Check sheet for the modelled part. Datum: model origin and axes. Units: mm. Face numbers are marked on the shaded views. A direction names the side the tool comes from. Coordinates: 2 decimals unless noted, no trailing zeros. Loops run counter-clockwise (first coordinate to the right, second up) from the corner with the lowest first, then second, coordinate; pieces in that order, holes last. Notation, with made-up numbers: (46.5, 41) - (91.5, 41) arc R9 ccw to (91.5, 46) - close; hole circle Ø11 at (78, -34). An arc over 180 degrees is marked (long way). Use a Markdown table: item, result. Add a question column.
1) Sectioned sample at B-B, the plane y = 7.5. Enter the section's corners in (x, z).
2) Thickness scan on line 1 (Z direction, x = 3.5, y = -6.25); line 2 (Y direction, x = -0.25, z = 61); line 3 (Z direction, x = 1.5, y = 1.75). Record the ranges inside material, lowest first.
3) Tool access check on the marked faces 1 and 2. Record the directions out of +Z, -Z, +X, -X, +Y, -Y that give a thin tool (end or side, any length) a straight path to the whole face; none if there is none.
4) Go/stop test with flat-tipped pins: P1, Ø1.5, axis at x = 2, y = 4, coming from the -Z side; P2, Ø6, axis at y = -1.5, z = 55, coming from the -X side. Record where each tip stops, or that it passes through.
5) Sectioned sample at A-A, the plane z = 31. Enter the section's corners in (x, y).
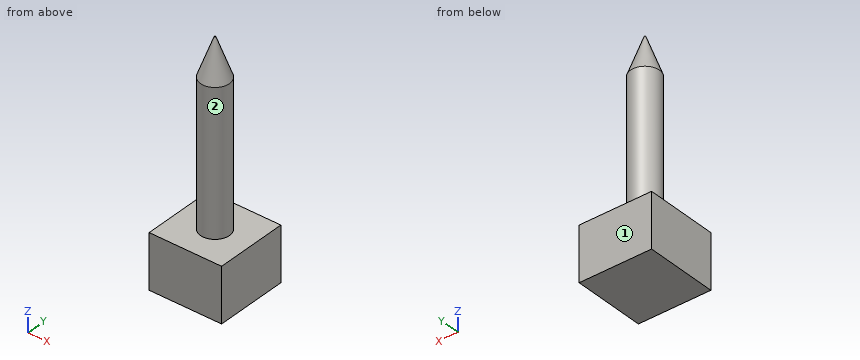
from build123d import *

# Parameters (mm, degrees)
SKETCH1_W           = 20
SKETCH1_H           = 20
BOSS_EXTRUDE1_DEPTH = 15
SKETCH2_R           = 4
BOSS_EXTRUDE2_DEPTH = 50
CHAMFER1_SIZE       = 10.5
CHAMFER1_SIZE2      = 3.82168746


with BuildPart() as part:
    # Sketch1 → Boss-Extrude1 (new body)
    with BuildSketch(Plane.XY):
        Rectangle(SKETCH1_W, SKETCH1_H)
    extrude(amount=BOSS_EXTRUDE1_DEPTH)

    # Sketch2 → Boss-Extrude2 (add)
    with BuildSketch(Plane.XY.offset(15)):
        Circle(SKETCH2_R)
    extrude(amount=BOSS_EXTRUDE2_DEPTH)

    # Chamfer1
    chamfer1_edges = [part.edges().sort_by_distance(p)[0] for p in [
        (-4, 0, 65),
    ]]
    chamfer1_side = [part.faces().sort_by_distance(p)[0] for p in [
        (-4, 0, 40),
    ]]
    chamfer(chamfer1_edges, length=CHAMFER1_SIZE, length2=CHAMFER1_SIZE2, reference=chamfer1_side[0])


solid = part.part
Solved:
| question | item | result |
|---|---|---|
| 1 | outline | (-10, 0) - (10, 0) - (10, 15) - (-10, 15) - close |
| 2 | line 1 | z = 0 to 15 |
| 2 | line 2 | y = -1.61 to 1.61 |
| 2 | line 3 | z = 0 to 59.16 |
| 3 | face 1 | +Z, -Z, +X, -X, +Y |
| 3 | face 2 | +Z |
| 4 | P1 | stops at z = 0 |
| 4 | P2 | stops at x = -4 |
| 5 | outline | circle Ø8 at (0, 0) |
